Read the model definition and answer for the solid it produces. Units are mm, in the model's axes. Face numbers are marked on the shaded views. Coordinates: 2 decimals unless noted, no trailing zeros. Order: outer loops, then holes, each group sorted by start corner. A loop starts at its lowest first (then second) coordinate and runs counter-clockwise, first axis right, second up. Notation, with made-up numbers: (-22.75, 57) -> (20.25, 57) arc R14 cw to (20.25, 69) -> close; hole circle Ø11 at (84, 5.25). An arc over 180 degrees is marked (long way). Answer as a JSON object with one key per item and string values. Group by question number.
1) Section A-A on z = 1121 is taken. Determine the outline of the cut face in (x, y).
2) Determine the mould class of the marked faces 1, 2 and 3 for opening direction Z: released by +Z, released by -Z, zero draft, split by the parting line, or undercut.
3) Consider L1, parallel to Y at x = -12, z = 1375; L2, parallel to Z at x = 228, y = 109.5; L3, parallel to Y at x = -90, z = 1045. Determine where each line is inside the solid, lowest interval first.
4) Given pin 1 (2 mm diameter, centred on y = 196.5, z = 1599.5, fed in from -X); pin 2 (1 mm diameter, centred on y = -90.5, z = 537.5, fed in from -X); pin 3 (6 mm diameter, centred on y = 131, z = 737, fed in from -X), each flat-ended and moving along its own axis, determine where each tip first touches the part or whether it passes through.
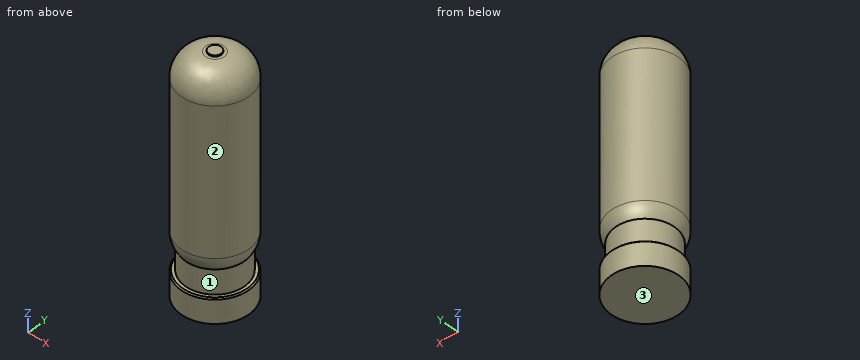
Autodesk Inventor part; units mm, degrees
ref_plane "YZ Plane" through (0, 0, 0) normal (1, 0, 0) x (0, 1, 0)
ref_plane "XZ Plane" through (0, 0, 0) normal (0, 1, 0) x (-1, 0, 0)
ref_plane "XY Plane" through (0, 0, 0) normal (0, 0, 1) x (1, 0, 0)
sketch "Sketch2" plane through (0, 0, 0) normal (0, 1, 0) x (-1, 0, 0)
  line L0 (0, 2130.997) -> (0, 0)
  line L1 (275, 1900) -> (75, 1900) construction
  line L2 (0, 1900) -> (0, 0)
  line L3 (0, 0) -> (275, 0)
  line L4 (275, 0) -> (275, 200)
  line L5 (275, 310) -> (75, 310) construction
  arc A0 (75, 310) -> (275, 510) centre (75, 510) ccw
  arc A1 (275, 1700) -> (75, 1900) centre (75, 1700) ccw
  line L6 (75, 1900) -> (0, 1900)
  line L7 (275, 1700) -> (275, 1900) construction
  line L8 (75, 310) -> (0, 310)
  line L9 (275, 310) -> (275, 510) construction
  line L10 (275, 510) -> (275, 1700)
  line L11 (275, 200) -> (240, 200)
  line L12 (240, 200) -> (240, 396.9735)
  line L13 (275, 200) -> (275, 310) construction
  line L14 (0, 1910) -> (50, 1910)
  line L15 (50, 1910) -> (50, 1900)
  point P0 (0, 1900)
  dimension "d3" = 550
  dimension "d7" = 200
  dimension "d8" = 200
  dimension "d9" = 35
  dimension "d10" = 200
  dimension "d12" = 50
  dimension "d13" = 10
  dimension "d14" = 1910
  dimension "d15" = 1600
revolve "Revolution1" add sketch "Sketch2" angle 360 about axis through (0, 0, 2130.997) along (0, 0, -1)
chamfer "Chamfer1" distance 10 angle 45 1 edges at (275, 0, 200)
equation "\"d3\" = D"
equation "\"d8\" = d7"
equation "\"d14\" = H1"
equation "\"d15\" = H2"
equation "\"H1\" = 1910"
equation "\"H2\" = 1600"
equation "\"D\" = 550"
properties part number "HY-H H2162–4T"
Worked answers:
{
 "1": {"outline": "circle Ø550 at (0, 0)"},
 "2": {"face 1": "undercut", "face 2": "zero draft", "face 3": "released by -Z"},
 "3": {"L1": "y = -274.74 to 274.74", "L2": "z = 0 to 200, 418.67 to 1791.33", "L3": "y = -259.86 to 259.86"},
 "4": {"pin 1": "stops at x = -193.4", "pin 2": "stops at x = -259.86", "pin 3": "stops at x = -243.39"}
}
